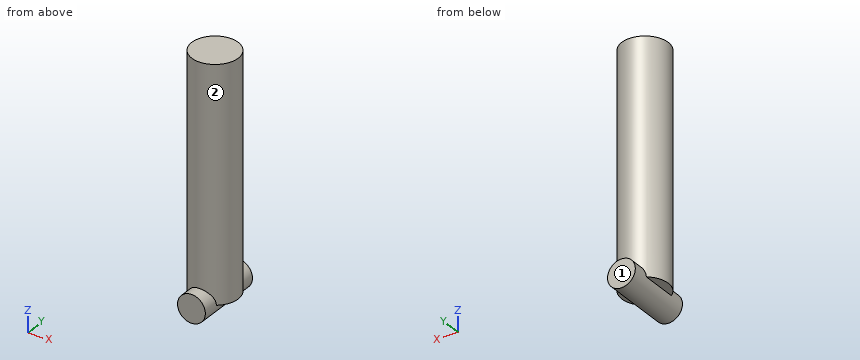
Autodesk Inventor part; units mm, degrees
ref_plane "作業平面1" through (0, 0, -300) normal (0, 0, 1) x (1, 0, 0)
sketch "スケッチ3" plane through (0, 0, 0) normal (0, 0, 1) x (1, 0, 0)
  circle A0 centre (0, 0) radius 25
  dimension "d7" = 50
extrude "押し出し2" add sketch "スケッチ3" against normal blind 300
sketch "スケッチ4" plane through (0, 0, 0) normal (1, 0, 0) x (0, 1, 0)
  line L0 (82.0674, 98.3645) -> (-82.6495, 98.3645)
  line L1 (-82.6495, 98.3645) -> (-82.6495, -50)
  line L2 (-82.6495, -50) -> (82.0674, -50)
  line L3 (82.0674, -50) -> (82.0674, 98.3645)
  line L4 (-115.5929, 0) -> (115.0108, 0)
  point P0 (0, 0)
  dimension "d10" = 50
extrude "押し出し3" cut sketch "スケッチ4" along normal mid plane 300
sketch "スケッチ5" plane through (0, 0, 0) normal (0, 1, 0) x (-1, 0, 0)
  circle A0 centre (0, -300) radius 15
  point P0 (0, 0)
  dimension "d13" = 30
  dimension "d14" = 300
extrude "押し出し4" add sketch "スケッチ5" along normal mid plane 75
properties part number "UpperlegP"
Geometry check sheet. Reference: the model listing, model coordinates, mm. Face numbers are marked on the shaded views. A direction names the side the tool comes from. Give positions to 0.01 mm unless a question says otherwise; leave off trailing zeros. Write each loop counter-clockwise with the first axis right and the second up, starting at its lowest first coordinate (ties: lowest second). Pieces come first, ordered by that corner, then holes.
1) Section check D-D, the plane z = -203.5. Record the boundary of the cut face in (x, y).
2) Section check B-B, the plane x = 0. Record the boundary of the cut face in (y, z), and give its area (3 significant figures).
3) Material ranges on L1, parallel to X at y = -1, z = -67; L2, parallel to X at y = 5, z = -79.5; L3, parallel to Z at x = -6, y = -16.5, recorded low to high.
4) Gauge pin test, flat ends, axial feed: pin 1 (8 mm diameter, centred on x = -20, y = 8.5, fed in from -Z); pin 2 (10 mm diameter, centred on y = 23, z = -162, fed in from +X); pin 3 (12 mm diameter, centred on x = 3.5, z = -102.5, fed in from +Y). Record the tip position at first contact, or that the pin passes through.
5) Section check A-A, the plane y = 0. Record the boundary of the cut face in (x, z), and give its area (3 significant figures).
6) Access from +Z, -Z, +X, -X, +Y, -Y to the whole of each face (thin tool, end or side, straight path). Record for the marked faces 1 and 2.
7) Section check C-C, the plane z = -291. Record the boundary of the cut face in (x, y).
Computed:
1. outline: circle Ø50 at (0, 0)
2. outline: (-37.5, -315) - (37.5, -315) - (37.5, -285) - (25, -285) - (25, -50) - (-25, -50) - (-25, -285) - (-37.5, -285) - close
2. area: 14,000 mm2
3. L1: x = -24.98 to 24.98
3. L2: x = -24.49 to 24.49
3. L3: z = -313.75 to -50
4. pin 1: stops at z = -300
4. pin 2: stops at x = 17.35
4. pin 3: stops at y = 25
5. outline: (-25, -300) - (-15, -300) arc R15 ccw to (15, -300) - (25, -300) - (25, -50) - (-25, -50) - close
5. area: 12,900 mm2
6. face 1: +Z, -Z, +X, -X, +Y
6. face 2: +Z
7. outline: (-12, -37.5) - (12, -37.5) - (12, -21.93) arc R25 ccw to (12, 21.93) - (12, 37.5) - (-12, 37.5) - (-12, 21.93) arc R25 ccw to (-12, -21.93) - close
